from build123d import *

# Parameters (mm, degrees)
SKETCH_1_R          = 2.25
EXTRUDE_1_DEPTH     = 6
SKETCH_2_R          = 1.02
CUT_EXTRUDE_1_DEPTH = 6
SKETCH_3_W          = 1
SKETCH_3_H          = 5
CUT_EXTRUDE_2_DEPTH = 2
CHAMFER_1_SIZE      = 0.25
CHAMFER_2_SIZE      = 0.25
CHAMFER_4_SIZE      = 0.25
CHAMFER_5_SIZE      = 0.1
CHAMFER_6_SIZE      = 0.1
CHAMFER_7_SIZE      = 0.1


with BuildPart() as part:
    # Эскиз1 → Бобышка-Вытянуть1 (new body)
    with BuildSketch(Plane.XY):
        Circle(SKETCH_1_R)
    extrude(amount=EXTRUDE_1_DEPTH)

    # Эскиз2 → Вырез-Вытянуть1 (cut)
    with BuildSketch(Plane.XY.offset(6)):
        Circle(SKETCH_2_R)
    extrude(amount=-CUT_EXTRUDE_1_DEPTH, mode=Mode.SUBTRACT)

    # Эскиз3 → Вырез-Вытянуть2 (cut)
    with BuildSketch(Plane.XY.offset(6)):
        Rectangle(SKETCH_3_W, SKETCH_3_H)
    extrude(amount=-CUT_EXTRUDE_2_DEPTH, mode=Mode.SUBTRACT)

    # Фаска1
    chamfer_1_edges = [part.edges().sort_by_distance(p)[0] for p in [
        (1.75890591, -1.40312152, 6),
    ]]
    chamfer(chamfer_1_edges, length=CHAMFER_1_SIZE)

    # Фаска2
    chamfer_2_edges = [part.edges().sort_by_distance(p)[0] for p in [
        (-2.25, 0, 6),
    ]]
    chamfer(chamfer_2_edges, length=CHAMFER_2_SIZE)

    # Фаска4
    chamfer_4_edges = [part.edges().sort_by_distance(p)[0] for p in [
        (-2.25, 0, 0),
    ]]
    chamfer(chamfer_4_edges, length=CHAMFER_4_SIZE)

    # Фаска5
    chamfer_5_edges = [part.edges().sort_by_distance(p)[0] for p in [
        (-1.02, 0, 0),
    ]]
    chamfer(chamfer_5_edges, length=CHAMFER_5_SIZE)

    # Фаска6
    chamfer_6_edges = [part.edges().sort_by_distance(p)[0] for p in [
        (0.880454428, -0.514975728, 6),
    ]]
    chamfer(chamfer_6_edges, length=CHAMFER_6_SIZE)

    # Фаска7
    chamfer_7_edges = [part.edges().sort_by_distance(p)[0] for p in [
        (-1.02, 0, 6),
    ]]
    chamfer(chamfer_7_edges, length=CHAMFER_7_SIZE)


solid = part.part
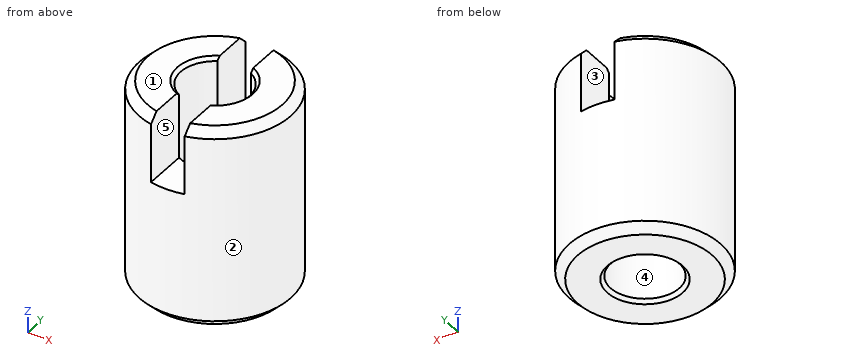
Could you check a few things on this model? Use its own coordinates, in mm. Face numbers are marked on the shaded views. A direction names the side the tool comes from. Give positions to 0.01 mm unless a question says otherwise; leave off trailing zeros. Loops run counter-clockwise (first coordinate to the right, second up) from the corner with the lowest first, then second, coordinate; pieces in that order, holes last. Notation, with made-up numbers: (25, -10.75) -> (31, -10.75) arc R11 ccw to (31, 6.25) -> close; hole circle Ø9 at (12.5, -6). An arc over 180 degrees is marked (long way). Answer as CSV lines item,"result". Start each with the question number.
(1) I need wall thicknesses on probe 1 along Y at (x, z) = (0, 2.1); probe 2 along Y at (x, z) = (-0.85, 1); probe 3 along X at (y, z) = (-0.75, 2.5). Which ranges of each line are inside material? Lowest first, please.
(2) We'd pull the mould along X, two halves only. Please class the marked faces 1, 2 and 3: released by +X, released by -X, zero draft, split by the parting line, or undercut.
(3) I'm going to push flat-ended pins straight in: pin 1 Ø0.7 at (y, z) = (1.5, 5) entering from +X; pin 2 Ø0.7 at (y, z) = (-2, 5.5) entering from +X; pin 3 Ø0.8 at (x, y) = (0, -1.5) entering from +Z. Where does each tip first touch, or does it pass through?
(4) If we section it at A-A on y = 0: Write out the boundary of the cut face in (x, z).
(5) If we section it at B-B on x = 0: Write out the boundary of the cut face in (y, z), then the cut area to 3 significant figures.
(6) If we section it at C-C on z = 3.5: Write out the boundary of the cut face in (x, y).
(7) Which directions (+Z, -Z, +X, -X, +Y, -Y) give clear straight access to the entire face, cutting with the end or side of a thin tool? Please do the marked faces 4 and 5.
Computed:
1,probe 1,"y = -2.25 to -1.02, 1.02 to 2.25"
1,probe 2,"y = -2.08 to -0.56, 0.56 to 2.08"
1,probe 3,"x = -2.12 to -0.69, 0.69 to 2.12"
2,face 1,"zero draft"
2,face 2,"split by the parting line"
2,face 3,"undercut"
3,pin 1,"stops at x = 1.93"
3,pin 2,"stops at x = 1.53"
3,pin 3,"stops at z = 4"
4,outline,"(-2.25, 0.25) -> (-2, 0) -> (-1.12, 0) -> (-1.02, 0.1) -> (-1.02, 5.9) -> (-1.12, 6) -> (-2, 6) -> (-2.25, 5.75) -> close; (1.02, 0.1) -> (1.12, 0) -> (2, 0) -> (2.25, 0.25) -> (2.25, 5.75) -> (2, 6) -> (1.12, 6) -> (1.02, 5.9) -> close"
5,outline,"(-2.25, 0.25) -> (-2, 0) -> (-1.12, 0) -> (-1.02, 0.1) -> (-1.02, 4) -> (-2.25, 4) -> close; (1.02, 0.1) -> (1.12, 0) -> (2, 0) -> (2.25, 0.25) -> (2.25, 4) -> (1.02, 4) -> close"
5,area,"9.77 mm2"
6,outline,"circle Ø4.5 at (0, 0); hole circle Ø2.04 at (0, 0)"
7,face 4,"+Z, -Z"
7,face 5,"+Z, +Y, -Y"
